Here's how the part is built. I have some questions about the finished solid (model axes, mm). A direction names the side the tool comes from. Round coordinates to 2 decimals unless told otherwise and drop trailing zeros. Loops run counter-clockwise (first coordinate to the right, second up) from the corner with the lowest first, then second, coordinate; pieces in that order, holes last. Notation, with made-up numbers: M 72.25,-14.5 L 94.25,-14.5 A31 ccw 94.25,17.5 Z; hole C 12,81.5 d7. An arc over 180 degrees is marked long. Answer as CSV lines item,"result".
Autodesk Fusion 360 part; units mm, degrees
sketch "Sketch1" plane through (0, 0, 0) normal (0, 1, 0) x (1, 0, 0)
  line L0 (25.6354, -40) -> (70.6354, -40)
  line L1 (80.6354, -30) -> (80.6354, 15)
  line L2 (80.6354, 15) -> (15.6354, 15)
  line L3 (15.6354, 15) -> (15.6354, -30)
  arc A0 (15.6354, -30) -> (25.6354, -40) centre (25.6354, -30) ccw
  arc A1 (70.6354, -40) -> (80.6354, -30) centre (70.6354, -30) ccw
  dimension "d1" = 65
  dimension "d2" = 55
  dimension "d3" = 10
  dimension "d4" = 10
extrude "Extrude2" add sketch "Sketch1" along normal blind 30
shell "Shell2" thickness 3 removed faces 1 at (58.9688, 20, -15)
sketch "Sketch2" plane through (0, 0, 0) normal (1, 0, 0) x (0, 1, 0)
  line L0 (21, 15.6496) -> (10, 15.6496)
  line L1 (10, 15.6496) -> (10, -16.8071)
  line L2 (10, -16.8071) -> (21, -16.8071)
  line L3 (21, -16.8071) -> (21, 15.6496)
  dimension "d11" = 11
extrude "Extrude3" cut sketch "Sketch2" along normal blind 25
1. I want a section at D-D, the plane y = 4.75. Please give me the cut outline in (x, z).
Evaluation:
outline,"M 15.64,-15 L 18.64,-15 L 18.64,30 A7 cw 25.64,37 L 70.64,37 A7 cw 77.64,30 L 77.64,-15 L 80.64,-15 L 80.64,30 A10 ccw 70.64,40 L 25.64,40 A10 ccw 15.64,30 Z"
2. We'd pull the mould along Y, two halves only. Please class faces 4 (the flat face through (17, 16, 15.65)), 5 (the flat face through (15.635, 8, 7)), 6 (the flat face through (48, 30, 12)): pulls with the +Y half, pulls with the -Y half, needs draft (parallel to the pull), parting line crosses it, or undercut.
Evaluation:
face 4,"undercut"
face 5,"needs draft"
face 6,"pulls with the +Y half"
3. I want a section at A-A, the plane z = 10. Please give me the cut outline in (x, y), and give its area (3 significant figures).
Evaluation:
outline,"M 15.64,0 L 80.64,0 L 80.64,30 L 15.64,30 L 15.64,21 L 18.64,21 L 18.64,27 L 77.64,27 L 77.64,3 L 18.64,3 L 18.64,10 L 15.64,10 Z"
area,"501 mm²"
4. I want a section at C-C, the plane x = 64.5. Please give me the cut outline in (y, z).
Evaluation:
outline,"M 0,-15 L 3,-15 L 3,37 L 27,37 L 27,-15 L 30,-15 L 30,40 L 0,40 Z"
5. For P1, Ø10, axis at x = 39.5, y = 16.5, coming from the -Z side; P2, Ø2.5, axis at x = 16.5, y = 17, coming from the -Z side, each with a flat end and sliding along its axis, tell me the tip position at first contact or that it passes through.
Evaluation:
P1,"stops at z = 37"
P2,"stops at z = 15.65"
6. If I drill on line 1 (X direction, y = 12.5, z = 19); line 2 (Y direction, x = 71, z = 3); line 3 (Z direction, x = 44, y = 10.75), over which ranges is the centre line in solid material (lowest first)? Write a range as [from, to].
Evaluation:
line 1,"x = [15.64, 18.64], [77.64, 80.64]"
line 2,"y = [0, 3], [27, 30]"
line 3,"z = [37, 40]"
7. Which directions (+Z, -Z, +X, -X, +Y, -Y) give clear straight access to the entire face, cutting with the end or side of a thin tool? Please do faces 1 (the flat face through (17, 10, 1)), 2 (the cylindrical face through (77.784, 14.79, 36.993)), 3 (the flat face through (48, 3, 11)).
Evaluation:
face 1,"-Z, -X"
face 2,"+Z, +X, +Y, -Y"
face 3,"-Z"
8. I want a section at B-B, the plane z = 21. Please give me the cut outline in (x, y).
Evaluation:
outline,"M 15.64,0 L 80.64,0 L 80.64,30 L 15.64,30 Z; hole M 18.64,3 L 77.64,3 L 77.64,27 L 18.64,27 Z"
